Check sheet for the modelled part. Datum: model origin and axes. Units: mm. Face numbers are marked on the shaded views. Round coordinates to 2 decimals unless told otherwise and drop trailing zeros. One line per question, with ' | ' between items.
```python
from build123d import *

# Parameters (mm, degrees)
SKETCH3_W                                           = 152.4
SKETCH3_H                                           = 22.225
BOSS_EXTRUDE1_DEPTH                                 = 76.2
FEET_R                                              = 6.35
RUBBER_FEET_DEPTH                                   = 3.175
CUT_EXTRUDE2_DEPTH                                  = 6.35
FILLET2_R                                           = 6.35
FILLET1_R                                           = 3.175
CBORE_FOR_M3_HEX_SOCKET_HEAD_CAP_SCREW1_D           = 3.6
CBORE_FOR_M3_HEX_SOCKET_HEAD_CAP_SCREW1_CBORE_D     = 6.5
CBORE_FOR_M3_HEX_SOCKET_HEAD_CAP_SCREW1_CBORE_DEPTH = 3.4
SKETCH10_R                                          = 38.1
CUT_EXTRUDE3_DEPTH                                  = 12.7


with BuildPart() as part:
    # Sketch3 → Boss-Extrude1 (new, symmetric)
    with BuildSketch(Plane.XY):
        Rectangle(SKETCH3_W, SKETCH3_H)
    extrude(amount=BOSS_EXTRUDE1_DEPTH, both=True)

    # Feet → Rubber Feet (cut)
    with BuildSketch(Plane.XZ.offset(11.1125)):
        with Locations(Location((-63.5, 63.5, 0), (0, 0, 270))):
            Circle(FEET_R)
        with Locations(Location((63.5, 63.5, 0), (0, 0, 90))):
            Circle(FEET_R)
        with Locations(Location((63.5, -63.5, 0), (0, 0, 270))):
            Circle(FEET_R)
        with Locations(Location((-63.5, -63.5, 0), (0, 0, 90))):
            Circle(FEET_R)
    extrude(amount=-RUBBER_FEET_DEPTH, mode=Mode.SUBTRACT)

    # Sketch6 → Cut-Extrude2 (cut)
    with BuildSketch(Plane(origin=(0, 11.1125, 0), x_dir=(1, 0, 0), z_dir=(0, 1, 0))):
        with BuildLine():
            Line((-63.5, -49.2125), (63.5, -49.2125))
            ThreePointArc((63.5, -49.2125), (71.4375, -57.15), (63.5, -65.0875))
            Line((63.5, -65.0875), (-63.5, -65.0875))
            ThreePointArc((-63.5, -65.0875), (-71.4375, -57.15), (-63.5, -49.2125))
        make_face()
    extrude(amount=-CUT_EXTRUDE2_DEPTH, mode=Mode.SUBTRACT)

    # Fillet2
    fillet2_edges = [part.edges().sort_by_distance(p)[0] for p in [
        (0, 4.7625, 49.2125),
        (71.4375, 4.7625, 57.15),
        (0, 4.7625, 65.0875),
        (-71.4375, 4.7625, 57.15),
    ]]
    fillet(fillet2_edges, radius=FILLET2_R - 0.0001)  # a hair under: the kernel refuses the full size

    # Fillet1
    fillet1_edges = [part.edges().sort_by_distance(p)[0] for p in [
        (76.2, 0, 76.2),
        (0, 11.1125, 76.2),
        (-76.2, 0, 76.2),
        (0, 11.1125, -76.2),
        (76.2, 0, -76.2),
        (0, -11.1125, -76.2),
        (-76.2, 0, -76.2),
        (0, -11.1125, 76.2),
        (-76.2, 11.1125, 0),
        (76.2, 11.1125, 0),
        (76.2, -11.1125, 0),
        (-76.2, -11.1125, 0),
    ]]
    fillet(fillet1_edges, radius=FILLET1_R)

    # CBORE for M3 Hex Socket Head Cap Screw1 (through all)
    with Locations(Plane(origin=(0, -11.1125, 0), x_dir=(-1, 0, 0), z_dir=(0, -1, 0))):
        with Locations((-50.8, -23.8125), (50.8, -23.8125)):
            CounterBoreHole(CBORE_FOR_M3_HEX_SOCKET_HEAD_CAP_SCREW1_D / 2, CBORE_FOR_M3_HEX_SOCKET_HEAD_CAP_SCREW1_CBORE_D / 2, CBORE_FOR_M3_HEX_SOCKET_HEAD_CAP_SCREW1_CBORE_DEPTH)

    # Sketch10 → Cut-Extrude3 (cut)
    with BuildSketch(Plane(origin=(0, 11.1125, 0), x_dir=(1, 0, 0), z_dir=(0, 1, 0))):
        with Locations(Location((0, 30.95625, 0), (0, 0, 270))):
            Circle(SKETCH10_R)
    extrude(amount=-CUT_EXTRUDE3_DEPTH, mode=Mode.SUBTRACT)

    # Sketch13 → CBORE for M3 Hex Socket Head Cap Screw2 (revolve, cut)
    with BuildSketch(Plane(origin=(0, -11.1125, -30.95625), x_dir=(0, 0, -1), z_dir=(1, 0, 0))):
        Polygon((0, 0), (0, 22.225), (1.8, 22.225), (1.8, 3.4), (3.25, 3.4), (3.25, 0.025), (3.275, 0), align=None)
    revolve(axis=Axis((0, -17.4625, -30.95625), (0, 1, 0)), mode=Mode.SUBTRACT)


solid = part.part
```
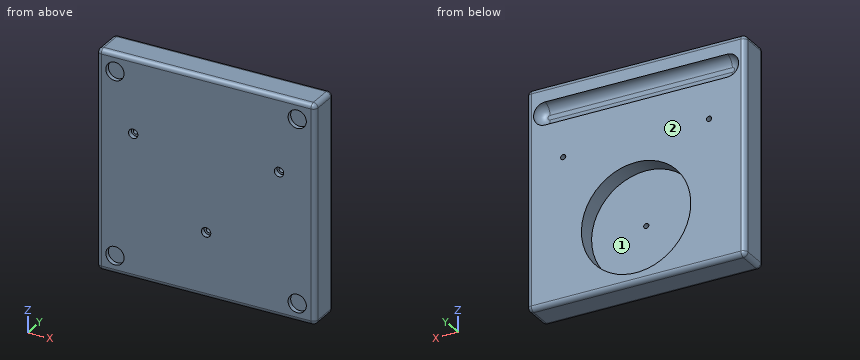
(1) Mould release check, pull along X, two halves, no side actions. Record for the marked faces 1 and 2: +X half, -X half, draft (parallel to the pull), parting line (faces both ways), or undercut.
Answer:
face 1: undercut | face 2: draft
(2) Go/stop test with flat-tipped pins: pin 1 (14.5 mm diameter, centred on x = 63.5, z = 63.5, fed in from -Y); pin 2 (7.5 mm diameter, centred on x = -63.5, z = 63.5, fed in from -Y); pin 3 (1.9 mm diameter, centred on x = 1.5, z = -32.5, fed in from -Y); pin 4 (8.5 mm diameter, centred on x = 0, z = -30.96, fed in from +Y). Record where each tip stops, or that it passes through.
Answer:
pin 1: stops at y = -11.11 | pin 2: stops at y = -7.94 | pin 3: stops at y = -7.71 | pin 4: stops at y = -1.59
(3) Scan lines: probe 1 along Z at (x, y) = (62.5, -8.5); probe 2 along X at (y, z) = (-9.75, -67); probe 3 along Y at (x, z) = (4.5, -67). Record each from-to range of solid material in increasing order.
Answer:
probe 1: z = -76.15 to -69.77, -57.23 to 57.23, 69.77 to 76.15 | probe 2: x = -75.63 to -68.8, -58.2 to 58.2, 68.8 to 75.63 | probe 3: y = -11.11 to -1.59
